The figure shows three views and two pictorial views of one solid part (mm, origin at its lowest corner). Answer the questions. A direction names the side the tool comes from. Give positions to 0.01 mm unless a question says otherwise; leave off trailing zeros. Order: outer loops, then holes, each group sorted by start corner. A loop starts at its lowest first (then second) coordinate and runs counter-clockwise, first axis right, second up. Notation, with made-up numbers: (39.25, -8.75) - (96.25, -8.75) arc R21 ccw to (96.25, 11.25) - close; hole circle Ø8 at (42, 39). An arc over 180 degrees is marked (long way). Answer as CSV lines item,"result". Start each with the question number.
1. Section C-C on z = 13.5 is taken. Give the vertices of the cut face in (x, y) (1 decimal), and give its area (3 significant figures).
2. Consider line 1 along X through (y, z) = (2, 19.05) (1 decimal); line 2 along Z through (x, y) = (15, 12) (1 decimal); line 3 along X through (y, z) = (11.55, 19.05). Determine where each line is inside the solid, lowest interval first. Write a range as [from, to].
3. Section A-A on x = 18 is taken. Count the separate pieces of the cut face and the enclosed holes in it, and give its area (3 significant figures).
4. Which of the six approach directions +Z, -Z, +X, -X, +Y, -Y give full straight-line access (tool end or side, diameter ignored) to the marked faces 5 and 6?
5. Determine the mould class of the marked faces 1, 2, 3 and 4 for opening direction Z: +Z half, -Z half, draft (parallel to the pull), parting line (faces both ways), or undercut.
6. Flat-ended cylindrical pins translate along their axes: pin 1 (6 mm diameter, centred on y = 7, z = 15.5, fed in from +X); pin 2 (6.5 mm diameter, centred on x = 20.5, z = 18.5, fed in from +Y) (3 decimals); pin 3 (4 mm diameter, centred on x = 10.5, y = 10.5, fed in from -Z); pin 4 (5.5 mm diameter, centred on x = 19.05, z = 19.05, fed in from +Y) (3 decimals). Find the tip coordinate at first contact, or state that the pin passes through.
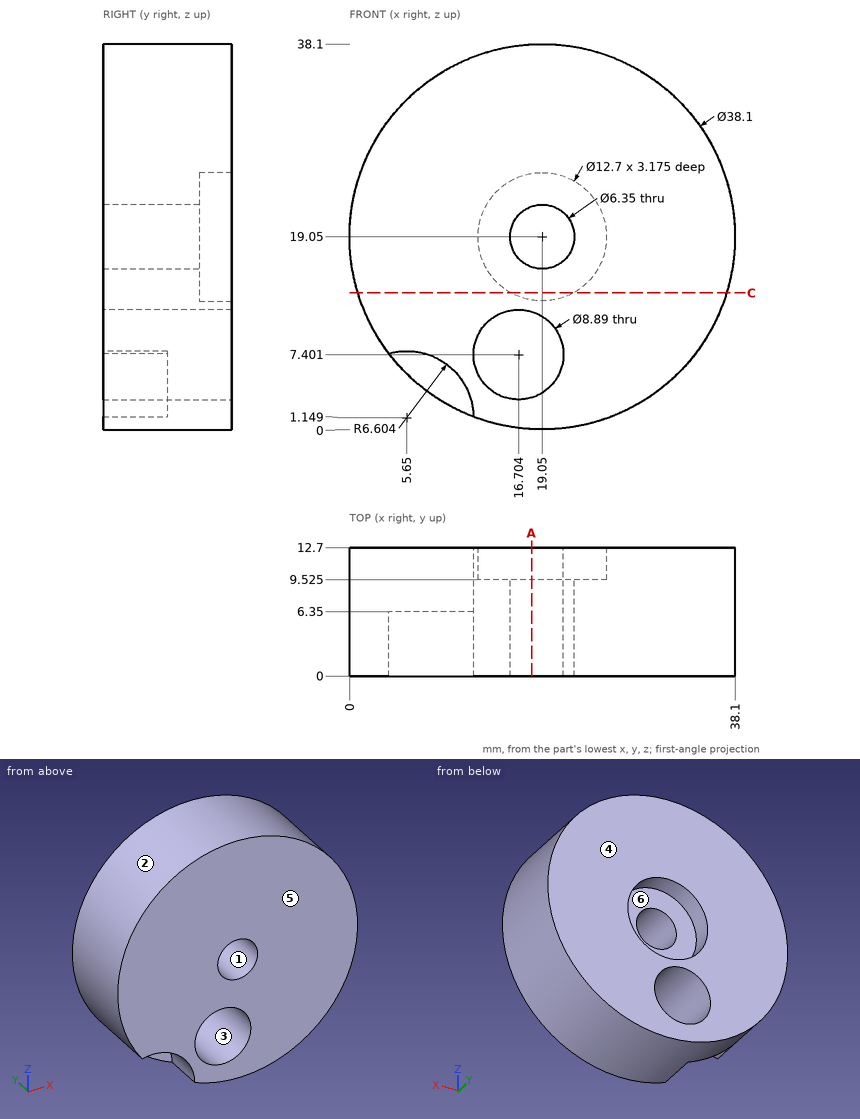
Checks:
1,outline,"(0.8, 0) - (37.3, 0) - (37.3, 12.7) - (22.1, 12.7) - (22.1, 9.5) - (16, 9.5) - (16, 12.7) - (0.8, 12.7) - close"
1,area,"443 mm²"
2,line 1,"x = [0, 15.9], [22.2, 38.1]"
2,line 2,"z = [0.4, 3.3], [11.5, 14.2], [23.9, 37.7]"
2,line 3,"x = [0, 12.7], [25.4, 38.1]"
3,separate pieces,"3"
3,enclosed holes,"0"
3,area,"278 mm²"
4,face 5,"+Z, -Z, +X, -X, -Y"
4,face 6,"+Y"
5,face 1,"undercut"
5,face 2,"parting line"
5,face 3,"undercut"
5,face 4,"draft"
6,pin 1,"stops at x = 38.09"
6,pin 2,"stops at y = 9.525"
6,pin 3,"stops at z = 1.16"
6,pin 4,"passes through"
